Autodesk Fusion 360 part; units mm, degrees
sketch "Sketch1" plane through (0, 0, 0) normal (0, 1, 0) x (1, 0, 0)
  line L0 (6.0101, -7) -> (-6.0101, -7)
  line L1 (-8.1, -12.8) -> (-8.1, -9.0899)
  line L2 (-6.0101, -7) -> (-8.1, -9.0899)
  line L3 (-4.1, -14.2) -> (-4.9, -14.2)
  line L4 (-4.9, -14.2) -> (-4.9, -15)
  line L5 (-4.1, -14.2) -> (-4.1, -12.8)
  line L6 (-13, -15) -> (-4.9, -15)
  line L7 (-8.1, -12.8) -> (-4.1, -12.8)
  line L8 (6.0101, -7) -> (8.1, -9.0899)
  line L9 (8.1, -12.8) -> (8.1, -9.0899)
  line L10 (8.1, -12.8) -> (4.1, -12.8)
  line L11 (4.1, -14.2) -> (4.1, -12.8)
  line L12 (4.1, -14.2) -> (4.9, -14.2)
  line L13 (4.9, -14.2) -> (4.9, -15)
  line L14 (13, -15) -> (4.9, -15)
  line L15 (14.2, -4.1) -> (14.2, -4.9)
  line L16 (12.8, -8.1) -> (9.0899, -8.1)
  line L17 (15, -13) -> (15, -4.9)
  line L18 (7, 6.0101) -> (9.0899, 8.1)
  line L19 (7, 6.0101) -> (7, -6.0101)
  line L20 (14.2, 4.9) -> (15, 4.9)
  line L21 (7, -6.0101) -> (9.0899, -8.1)
  line L22 (14.2, -4.1) -> (12.8, -4.1)
  line L23 (14.2, 4.1) -> (12.8, 4.1)
  line L24 (15, 13) -> (15, 4.9)
  line L25 (14.2, -4.9) -> (15, -4.9)
  line L26 (12.8, 8.1) -> (9.0899, 8.1)
  line L27 (12.8, 8.1) -> (12.8, 4.1)
  line L28 (12.8, -8.1) -> (12.8, -4.1)
  line L29 (14.2, 4.1) -> (14.2, 4.9)
  line L30 (4.1, 14.2) -> (4.9, 14.2)
  line L31 (8.1, 12.8) -> (8.1, 9.0899)
  line L32 (13, 15) -> (4.9, 15)
  line L33 (-6.0101, 7) -> (-8.1, 9.0899)
  line L34 (-6.0101, 7) -> (6.0101, 7)
  line L35 (-4.9, 14.2) -> (-4.9, 15)
  line L36 (6.0101, 7) -> (8.1, 9.0899)
  line L37 (4.1, 14.2) -> (4.1, 12.8)
  line L38 (-4.1, 14.2) -> (-4.1, 12.8)
  line L39 (-13, 15) -> (-4.9, 15)
  line L40 (4.9, 14.2) -> (4.9, 15)
  line L41 (-8.1, 12.8) -> (-8.1, 9.0899)
  line L42 (-8.1, 12.8) -> (-4.1, 12.8)
  line L43 (8.1, 12.8) -> (4.1, 12.8)
  line L44 (-4.1, 14.2) -> (-4.9, 14.2)
  line L45 (-14.2, 4.1) -> (-14.2, 4.9)
  line L46 (-12.8, 8.1) -> (-9.0899, 8.1)
  line L47 (-15, 13) -> (-15, 4.9)
  line L48 (-7, -6.0101) -> (-9.0899, -8.1)
  line L49 (-7, -6.0101) -> (-7, 6.0101)
  line L50 (-14.2, -4.9) -> (-15, -4.9)
  line L51 (-7, 6.0101) -> (-9.0899, 8.1)
  line L52 (-14.2, 4.1) -> (-12.8, 4.1)
  line L53 (-14.2, -4.1) -> (-12.8, -4.1)
  line L54 (-15, -13) -> (-15, -4.9)
  line L55 (-14.2, 4.9) -> (-15, 4.9)
  line L56 (-12.8, -8.1) -> (-9.0899, -8.1)
  line L57 (-12.8, -8.1) -> (-12.8, -4.1)
  line L58 (-12.8, 8.1) -> (-12.8, 4.1)
  line L59 (-14.2, -4.1) -> (-14.2, -4.9)
  circle A0 centre (0, 0) radius 5
  circle A1 centre (-11.55, -11.55) radius 2.25
  circle A2 centre (11.55, -11.55) radius 2.25
  circle A3 centre (11.55, 11.55) radius 2.25
  circle A4 centre (-11.55, 11.55) radius 2.25
  arc A5 (-15, -13) -> (-13, -15) centre (-13, -13) ccw
  arc A6 (13, -15) -> (15, -13) centre (13, -13) ccw
  arc A7 (15, 13) -> (13, 15) centre (13, 13) ccw
  arc A8 (-13, 15) -> (-15, 13) centre (-13, 13) ccw
  dimension "d17" = 10
  dimension "d22" = 4.5
  dimension "d24" = 360
  dimension "d25" = 2
extrude "Extrude1" add sketch "Sketch1" along normal blind 500
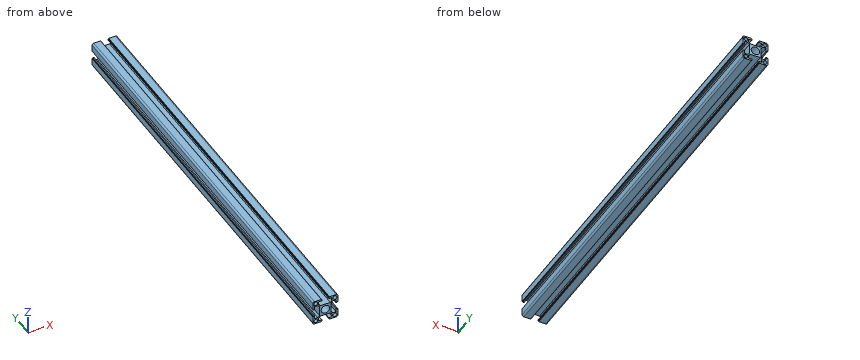
For this review, take the finished solid that the model builds, in its own axes (mm). Give positions to 0.01 mm unless a question says otherwise; leave off trailing zeros. Loops run counter-clockwise (first coordinate to the right, second up) from the corner with the lowest first, then second, coordinate; pieces in that order, holes last.
Item 1: Insertion check: pin 1 (3.5 mm diameter, centred on x = 11.55, z = 11.55, fed in from +Y); pin 2 (6 mm diameter, centred on x = 1, y = 328, fed in from -Z). Each pin has a flat end and moves straight along its axis. Give the tip position at first contact, or say it passes through.
Item 2: Take a section at A-A, the plane x = 0. State the section outline as (y, z) points, and give its area (3 significant figures).
Item 3: Take a section at C-C, the plane y = 62. Give the number of separate pieces and of enclosed holes in the cut face, and give its area (3 significant figures).
Item 4: Take a section at B-B, the plane z = 0. State the section outline as (x, y) points.
Item 5: For line 1 along X through (y, z) = (348, -11.55); line 2 along X through (y, z) = (96, -10.25), list the stretches that pass through material, from the lowest coordinate up.
Calculated:
1. pin 1: passes through
1. pin 2: stops at z = -7
2. outline: (0, -7) - (500, -7) - (500, -5) - (0, -5) - close; (0, 5) - (500, 5) - (500, 7) - (0, 7) - close
2. area: 2,000 mm2
3. separate pieces: 1
3. enclosed holes: 5
3. area: 319 mm2
4. outline: (-7, 0) - (-5, 0) - (-5, 500) - (-7, 500) - close; (5, 0) - (7, 0) - (7, 500) - (5, 500) - close
5. line 1: x = -15 to -13.8, -9.3 to -8.1, 8.1 to 9.3, 13.8 to 15
5. line 2: x = -15 to -13.39, -9.71 to -8.1, 8.1 to 9.71, 13.39 to 15
